The model under review builds one solid part; all positions refer to its coordinate system, in mm. A direction names the side the tool comes from. Give positions to 0.01 mm unless a question says otherwise; leave off trailing zeros. Loops run counter-clockwise (first coordinate to the right, second up) from the corner with the lowest first, then second, coordinate; pieces in that order, holes last. Notation, with made-up numbers: M 73,-35 L 90,-35 A14 ccw 90,-21 Z; hole C 38,27.25 d4. An arc over 180 degrees is marked long. Write item = value, one per line. Start each with the question number.
1. We need section B-B on x = -51. Give the boundary of the cut face in (y, z), then the cut area to 3 significant figures.
2. For pin 1 (1.5 mm diameter, centred on x = -49, y = -0.5, fed in from -Z); pin 2 (2 mm diameter, centred on y = 0.5, z = 15, fed in from -X), all flat-tipped, find the tip position at first contact; note any pin that passes through.
3. We need section A-A on y = 0.2. Give the boundary of the cut face in (x, z), then the cut area to 3 significant figures.
4. Wall thickness on line 1 along X through (y, z) = (-1.15, 20); line 2 along Z through (x, y) = (-28.5, 0.15): over which ranges is each line inside the solid? List them lowest first. Write a range as from..to.
5. For faces 1 (the face through (19, 0, 0)), 2 (the face through (-24, 0, 12)), list the 3-axis set-ups (+Z, -Z, +X, -X, +Y, -Y) from which the entire face can be reached by the end or side of a thin tool; tool diameter is ignored.
6. We need section C-C on z = 6. Give the boundary of the cut face in (x, y).
Autodesk Inventor part; units mm, degrees
ref_plane "YZ Plane" through (0, 0, 0) normal (1, 0, 0) x (0, 1, 0)
ref_plane "XZ Plane" through (0, 0, 0) normal (0, 1, 0) x (-1, 0, 0)
ref_plane "XY Plane" through (0, 0, 0) normal (0, 0, 1) x (1, 0, 0)
sketch "Sketch2" plane through (0, 0, 0) normal (0, 0, 1) x (1, 0, 0)
  line L0 (-64, -2) -> (64, -2)
  line L1 (64, -2) -> (64, 2)
  line L2 (64, 2) -> (-64, 2)
  line L3 (-64, 2) -> (-64, -2)
  line L4 (-64, -2) -> (64, 2) construction
  line L5 (64, -2) -> (-64, 2) construction
  point P0 (0, 0)
  dimension "d0" = 4
  dimension "d1" = 128
extrude "Extrusion1" add sketch "Sketch2" along normal blind 55
sketch "Sketch3" plane through (-64, -2, 0) normal (0, -1, 0) x (1, 0, 0)
  line L0 (0, 0) -> (128, 0)
  line L1 (0, 0) -> (40, 0)
  line L2 (40, 0) -> (40, 25)
  line L3 (40, 25) -> (0, 25)
  line L4 (0, 25) -> (0, 0)
  point P0 (64, 0)
  dimension "d4" = 40
  dimension "d5" = 25
extrude "Extrusion2" cut sketch "Sketch3" against normal through all
properties part number "divider"
Final values:
q1.outline = M -2,25 L 2,25 L 2,55 L -2,55 Z
q1.area = 120 mm²
q2.pin_1 = 25
q2.pin_2 = -24
q3.outline = M -64,25 L -24,25 L -24,0 L 64,0 L 64,55 L -64,55 Z
q3.area = 6,040 mm²
q4.line_1 = -24..64
q4.line_2 = 25..55
q5.face_1 = -Z, +X, -X, +Y, -Y
q5.face_2 = -Z, -X, +Y, -Y
q6.outline = M -24,-2 L 64,-2 L 64,2 L -24,2 Z
